The listing builds one solid part. Answer for the finished solid, in the listing's coordinates (mm). A direction names the side the tool comes from. Coordinates: 2 decimals unless noted, no trailing zeros. Loops run counter-clockwise (first coordinate to the right, second up) from the corner with the lowest first, then second, coordinate; pieces in that order, holes last. Notation, with made-up numbers: M -20,7 L -6,7 A23 ccw -6,35 Z; hole C -9.75,40.5 d9. An arc over 180 degrees is marked long. Return JSON: item names as keys, results as strings. Group by question number.
1. Section A-A (x = 0) is taken. Write down the section's boundary in (y, z).
2. Section D-D (x = 31) is taken. Write down the section's boundary in (y, z).
3. The mould has two halves that part along Y. Classify faces 4 (the face through (5.43, -26.25, 1.48)), 5 (the face through (-27.038, -7.581, 1.479)), 6 (the face through (0.22, -45.56, 1.48)), 7 (the face through (0, -3, 0)): pulls with the +Y half, pulls with the -Y half, needs draft (parallel to the pull), parting line crosses it, or undercut.
4. Section B-B (y = 0) is taken. Write down the section's boundary in (x, z), then the cut area to 3 significant figures.
5. Given P1, Ø6.5, axis at x = 0, y = -35.56, coming from the +Z side; P2, Ø1.5, axis at x = -36, z = 1.5, coming from the +Y side; P3, Ø1, axis at y = -18.5, z = 2.5, coming from the -X side, each flat-ended and moving along its own axis, determine where each tip first touches the part or whether it passes through.
6. Which of the six approach directions +Z, -Z, +X, -X, +Y, -Y give full straight-line access (tool end or side, diameter ignored) to faces 1 (the face through (16.45, -19.16, 1.48)), 2 (the face through (-45.354, -9.314, 1.479)), 3 (the face through (-1, 4, 1))?
7. Section C-C (z = 0.85) is taken. Write down the section's boundary in (x, y), then the cut area to 3 significant figures.
8. Straight lines are drawn through the part: L1, parallel to Y at x = 0, z = 0.7; L2, parallel to X at y = -1.5, z = 1.5; L3, parallel to Y at x = 4.5, z = 1.2. For each, find the intervals that lie inside material, in ascending order. Write a range as from..to.
```python
from build123d import *

# Parameters (mm, degrees)
SKETCH_1_R      = 3.5
EXTRUDE_2_DEPTH = 3


with BuildPart() as part:
    # 草圖1 → 填料-伸長2 (new body)
    with BuildSketch(Plane.XY):
        with BuildLine():
            Line((43.25190796, -10.159525413), (12.124130277, -31.955429995))
            ThreePointArc((12.124130277, -31.955429995), (10.595221, -33.670386808), (9.994674972, -35.888039829))
            ThreePointArc((9.994674972, -35.888039829), (0, -45.561739054), (-9.994674972, -35.888039829))
            ThreePointArc((-9.994674972, -35.888039829), (-10.595221, -33.670386808), (-12.124130277, -31.955429995))
            Line((-12.124130277, -31.955429995), (-43.25190796, -10.159525413))
            ThreePointArc((-43.25190796, -10.159525413), (-45.386357993, -9.309370423), (-47.67566901, -9.503523757))
            ThreePointArc((-47.67566901, -9.503523757), (-60.324596253, 3.007057995), (-42.787426746, 6))
            ThreePointArc((-42.787426746, 6), (-41.023494723, 4.527864045), (-38.787426746, 4))
            Line((-38.787426746, 4), (38.787426746, 4))
            ThreePointArc((38.787426746, 4), (41.023494723, 4.527864045), (42.787426746, 6))
            ThreePointArc((42.787426746, 6), (60.324596253, 3.007057995), (47.67566901, -9.503523757))
            ThreePointArc((47.67566901, -9.503523757), (45.386357993, -9.309370423), (43.25190796, -10.159525413))
        make_face()
        with Locations((50.787426746, 0)):
            Circle(SKETCH_1_R, mode=Mode.SUBTRACT)
        with Locations((-50.787426746, 0)):
            Circle(SKETCH_1_R, mode=Mode.SUBTRACT)
        with Locations((0, -35.561739054)):
            Circle(SKETCH_1_R, mode=Mode.SUBTRACT)
        with BuildLine():
            Line((-22.243073525, -4), (22.243073525, -4))
            ThreePointArc((22.243073525, -4), (27.011658278, -7.496471002), (25.110955706, -13.095760221))
            Line((25.110955706, -13.095760221), (7.535518786, -25.40221364))
            ThreePointArc((7.535518786, -25.40221364), (5.401068753, -26.252368631), (3.111757736, -26.058215297))
            ThreePointArc((3.111757736, -26.058215297), (0, -25.561739054), (-3.111757736, -26.058215297))
            ThreePointArc((-3.111757736, -26.058215297), (-5.401068753, -26.252368631), (-7.535518786, -25.40221364))
            Line((-7.535518786, -25.40221364), (-25.110955706, -13.095760221))
            ThreePointArc((-25.110955706, -13.095760221), (-27.011658278, -7.496471002), (-22.243073525, -4))
        make_face(mode=Mode.SUBTRACT)
    extrude(amount=EXTRUDE_2_DEPTH)


solid = part.part
```
Worked out:
{
 "1": {"outline": "M -45.56,0 L -39.06,0 L -39.06,3 L -45.56,3 Z; M -32.06,0 L -25.56,0 L -25.56,3 L -32.06,3 Z; M -4,0 L 4,0 L 4,3 L -4,3 Z"},
 "2": {"outline": "M -18.74,0 L 4,0 L 4,3 L -18.74,3 Z"},
 "3": {"face 4": "undercut", "face 5": "undercut", "face 6": "pulls with the -Y half", "face 7": "needs draft"},
 "4": {"outline": "M -60.79,0 L -54.29,0 L -54.29,3 L -60.79,3 Z; M -47.29,0 L 47.29,0 L 47.29,3 L -47.29,3 Z; M 54.29,0 L 60.79,0 L 60.79,3 L 54.29,3 Z", "area": "323 mm^2"},
 "5": {"P1": "through", "P2": "y = 4", "P3": "x = -32.05"},
 "6": {"face 1": "+Z, -Z", "face 2": "+Z, -Z, -Y", "face 3": "+Z, -Z, +Y"},
 "7": {"outline": "M -47.68,-9.5 A5 cw -43.25,-10.16 L -12.12,-31.96 A5 cw -9.99,-35.89 A10 ccw 9.99,-35.89 A5 cw 12.12,-31.96 L 43.25,-10.16 A5 cw 47.68,-9.5 A10 ccw long 42.79,6 A5 cw 38.79,4 L -38.79,4 A5 cw -42.79,6 A10 ccw long Z; hole C -50.79,0 d7; hole M -25.11,-13.1 L -7.54,-25.4 A5 ccw -3.11,-26.06 A10 cw 3.11,-26.06 A5 ccw 7.54,-25.4 L 25.11,-13.1 A5 ccw 22.24,-4 L -22.24,-4 A5 ccw Z; hole C 0,-35.56 d7; hole C 50.79,0 d7", "area": "2,260 mm^2"},
 "8": {"L1": "-45.56..-39.06, -32.06..-25.56, -4..4", "L2": "-60.67..-53.95, -47.63..47.63, 53.95..60.67", "L3": "-44.49..-26.3, -4..4"}
}
